Work out the finished part from the listing and answer in its coordinate system (mm). A direction names the side the tool comes from. Round coordinates to 2 decimals unless told otherwise and drop trailing zeros. Write each loop counter-clockwise with the first axis right and the second up, starting at its lowest first coordinate (ties: lowest second). Pieces come first, ordered by that corner, then holes. Notation, with made-up numbers: M 15,71.25 L 71,71.25 A10 ccw 71,84.25 Z; hole C 83.5,55.5 d10. An arc over 180 degrees is marked long. Answer in a Markdown table with one row per item.
```python
from build123d import *

# Parameters (mm, degrees)
SKETCH001_W     = 212.5
SKETCH001_H     = 62.8
PAD_DEPTH       = 1.5
SKETCH_W        = 12.5
SKETCH_H        = 12.5
POCKET_DEPTH    = 1
SKETCH002_W     = 6
SKETCH002_H     = 1.5
POCKET001_DEPTH = 1.501
SKETCH003_R     = 2
SKETCH003_R_2   = 1
PAD001_DEPTH    = 7
SKETCH004_R     = 1
POCKET002_DEPTH = 1.4
FILLET_R        = 3


with BuildPart() as part:
    # Sketch001 → Pad (new body)
    with BuildSketch(Plane.XY):
        with Locations((90, 15)):
            Rectangle(SKETCH001_W, SKETCH001_H)
    extrude(amount=-PAD_DEPTH)

    # Sketch → Pocket (cut)
    with BuildSketch(Plane.XY):
        Rectangle(SKETCH_W, SKETCH_H)
        with Locations((30, 0)):
            Rectangle(SKETCH_W, SKETCH_H)
        with Locations((60, 0)):
            Rectangle(SKETCH_W, SKETCH_H)
        with Locations((90, 0)):
            Rectangle(SKETCH_W, SKETCH_H)
        with Locations((120, 0)):
            Rectangle(SKETCH_W, SKETCH_H)
        with Locations((150, 0)):
            Rectangle(SKETCH_W, SKETCH_H)
        with Locations((180, 0)):
            Rectangle(SKETCH_W, SKETCH_H)
        with Locations((15, 30)):
            Rectangle(SKETCH_W, SKETCH_H)
        with Locations((45, 30)):
            Rectangle(SKETCH_W, SKETCH_H)
        with Locations((105, 30)):
            Rectangle(SKETCH_W, SKETCH_H)
        with Locations((135, 30)):
            Rectangle(SKETCH_W, SKETCH_H)
        with Locations((165, 30)):
            Rectangle(SKETCH_W, SKETCH_H)
    extrude(amount=-POCKET_DEPTH, mode=Mode.SUBTRACT)

    # Sketch002 (on Face4 of Pocket) → Pocket001 (cut, through all)
    with BuildSketch(Plane.XY):
        with Locations((180, 7)):
            Rectangle(SKETCH002_W, SKETCH002_H)
        with Locations((180, -7)):
            Rectangle(SKETCH002_W, SKETCH002_H)
        with Locations((150, -7)):
            Rectangle(SKETCH002_W, SKETCH002_H)
        with Locations((150, 7)):
            Rectangle(SKETCH002_W, SKETCH002_H)
        with Locations((120, -7)):
            Rectangle(SKETCH002_W, SKETCH002_H)
        with Locations((120, 7)):
            Rectangle(SKETCH002_W, SKETCH002_H)
        with Locations((90, -7)):
            Rectangle(SKETCH002_W, SKETCH002_H)
        with Locations((90, 7)):
            Rectangle(SKETCH002_W, SKETCH002_H)
        with Locations((60, -7)):
            Rectangle(SKETCH002_W, SKETCH002_H)
        with Locations((60, 7)):
            Rectangle(SKETCH002_W, SKETCH002_H)
        with Locations((90, -7)):
            Rectangle(SKETCH002_W, SKETCH002_H)
        with Locations((90, 7)):
            Rectangle(SKETCH002_W, SKETCH002_H)
        with Locations((60, -7)):
            Rectangle(SKETCH002_W, SKETCH002_H)
        with Locations((60, 7)):
            Rectangle(SKETCH002_W, SKETCH002_H)
        with Locations((165, 37)):
            Rectangle(SKETCH002_W, SKETCH002_H)
        with Locations((165, 23)):
            Rectangle(SKETCH002_W, SKETCH002_H)
        with Locations((135, 37)):
            Rectangle(SKETCH002_W, SKETCH002_H)
        with Locations((135, 23)):
            Rectangle(SKETCH002_W, SKETCH002_H)
        with Locations((30, 7)):
            Rectangle(SKETCH002_W, SKETCH002_H)
        with Locations((30, -7)):
            Rectangle(SKETCH002_W, SKETCH002_H)
        with Locations((0, 7)):
            Rectangle(SKETCH002_W, SKETCH002_H)
        with Locations((0, -7)):
            Rectangle(SKETCH002_W, SKETCH002_H)
        with Locations((105, 37)):
            Rectangle(SKETCH002_W, SKETCH002_H)
        with Locations((105, 23)):
            Rectangle(SKETCH002_W, SKETCH002_H)
        with Locations((45, 37)):
            Rectangle(SKETCH002_W, SKETCH002_H)
        with Locations((45, 23)):
            Rectangle(SKETCH002_W, SKETCH002_H)
        with Locations((15, 23)):
            Rectangle(SKETCH002_W, SKETCH002_H)
        with Locations((15, 37)):
            Rectangle(SKETCH002_W, SKETCH002_H)
    extrude(amount=-POCKET001_DEPTH, mode=Mode.SUBTRACT)

    # Sketch003 (on Face4 of Pocket001) → Pad001 (join)
    with BuildSketch(Plane.XY):
        with Locations((-11.25, 41.4)):
            Circle(SKETCH003_R)
        with Locations((-11.25, 41.4)):
            Circle(SKETCH003_R_2, mode=Mode.SUBTRACT)
        with Locations((-11.25, -11.4)):
            Circle(SKETCH003_R)
        with Locations((-11.25, -11.4)):
            Circle(SKETCH003_R_2, mode=Mode.SUBTRACT)
        with Locations((191.25, -11.4)):
            Circle(SKETCH003_R)
        with Locations((191.25, -11.4)):
            Circle(SKETCH003_R_2, mode=Mode.SUBTRACT)
        with Locations((191.25, 41.4)):
            Circle(SKETCH003_R)
        with Locations((191.25, 41.4)):
            Circle(SKETCH003_R_2, mode=Mode.SUBTRACT)
    extrude(amount=PAD001_DEPTH)

    # Sketch004 (on Face4 of Pad001) → Pocket002 (cut)
    with BuildSketch(Plane.XY):
        with Locations((-11.25, -1.25)):
            Circle(SKETCH004_R)
        with Locations((-11.25, 31.25)):
            Circle(SKETCH004_R)
        with Locations((191.25, 31.25)):
            Circle(SKETCH004_R)
        with Locations((191.25, -1.25)):
            Circle(SKETCH004_R)
    extrude(amount=-POCKET002_DEPTH, mode=Mode.SUBTRACT)

    # Fillet
    fillet_edges = [part.edges().sort_by_distance(p)[0] for p in [
        (196.25, 46.4, -0.75),
        (196.25, -16.4, -0.75),
        (-16.25, -16.4, -0.75),
        (-16.25, 46.4, -0.75),
    ]]
    fillet(fillet_edges, radius=FILLET_R)


solid = part.part
```
1. A tool of negligible diameter and unlimited length cuts with its end or side. For faces 3 (the flat face through (190, 41, 7)), 4 (the flat face through (135, 30, -1)), from which of +Z, -Z, +X, -X, +Y, -Y can it reach the whole face along a straight path? Write none if from no direction.
Calculated:
| item | result |
|---|---|
| face 3 | +Z, +X, -X, +Y, -Y |
| face 4 | +Z |
2. The part is cut by section A-A (z = 4.25). Determine the outline of the cut face in (x, y), plus the area to 3 significant figures.
Calculated:
| item | result |
|---|---|
| outline | C -11.25,-11.4 d4; C -11.25,41.4 d4; C 191.25,-11.4 d4; C 191.25,41.4 d4; hole C -11.25,-11.4 d2; hole C -11.25,41.4 d2; hole C 191.25,-11.4 d2; hole C 191.25,41.4 d2 |
| area | 37.7 mm² |
3. The part is cut by section B-B (x = 45). Determine the outline of the cut face in (y, z), plus the area to 3 significant figures.
Calculated:
| item | result |
|---|---|
| outline | M -16.4,-1.5 L 22.25,-1.5 L 22.25,0 L -16.4,0 Z; M 23.75,-1.5 L 36.25,-1.5 L 36.25,-1 L 23.75,-1 Z; M 37.75,-1.5 L 46.4,-1.5 L 46.4,0 L 37.75,0 Z |
| area | 77.2 mm² |
4. Consider line 1 along Y through (x, z) = (-11.25, 4.75); line 2 along Y through (x, z) = (-11.25, -0.75); line 3 along Z through (x, y) = (-6, 16.5). Determine where each line is inside the solid, lowest interval first. Write a range as from..to.
Calculated:
| item | result |
|---|---|
| line 1 | y = -13.4..-12.4, -10.4..-9.4, 39.4..40.4, 42.4..43.4 |
| line 2 | y = -16.4..-2.25, -0.25..30.25, 32.25..46.4 |
| line 3 | z = -1.5..0 |
5. The part is cut by section D-D (x = 71). Determine the outline of the cut face in (y, z), plus the area to 3 significant figures.
Calculated:
| item | result |
|---|---|
| outline | M -16.4,-1.5 L 46.4,-1.5 L 46.4,0 L -16.4,0 Z |
| area | 94.2 mm² |
6. Given pin 1 (4 mm diameter, centred on y = 13, z = 1.5, fed in from +X); pin 2 (3 mm diameter, centred on y = 4, z = 2, fed in from -X), each flat-ended and moving along its own axis, determine where each tip first touches the part or whether it passes through.
Calculated:
| item | result |
|---|---|
| pin 1 | stops at x = 196.25 |
| pin 2 | passes through |
7. Determine the mould class of faces 1 (the cylindrical face through (-11.684, 39.448, 3.451)), 2 (the flat face through (-11, -10, 7)) for opening direction X: released by +X, released by -X, zero draft, split by the parting line, or undercut.
Calculated:
| item | result |
|---|---|
| face 1 | undercut |
| face 2 | zero draft |
